```python
from build123d import *

# Parameters (mm, degrees)
F1_DEPTH = 27
F2_W     = 1
F2_H     = 14.5
F2_W_2   = 1.25
F2_H_2   = 3
F2_H_3   = 4.5
F3_DEPTH = 75
F4_R     = 2


with BuildPart() as f1:
    # F0 (on Top) → F1 (new body)
    with BuildSketch(Plane.XY):
        Polygon((10, -5), (27, -5), (27, 5), (-27, 5), (-27, -5), (-10, -5), (-10, -2.5), (10, -2.5), align=None)
    extrude(amount=F1_DEPTH)

    # F2 (on face) → F3 (cut)
    with BuildSketch(Plane(origin=(-27, 0, 0), x_dir=(0, -1, 0), z_dir=(-1, 0, 0))):
        with Locations((-4.5, 12.25)):
            Rectangle(F2_W, F2_H)
        with Locations((-3.375, 12.25)):
            Rectangle(F2_W_2, F2_H)
        with Locations((-4.5, 3.5)):
            Rectangle(F2_W, F2_H_2)
        with Locations((-4.5, 21.75)):
            Rectangle(F2_W, F2_H_3)
    extrude(amount=-F3_DEPTH, mode=Mode.SUBTRACT)

    # F4
    f4_edges = [f1.edges().sort_by_distance(p)[0] for p in [
        (0, 5, 27),
    ]]
    fillet(f4_edges, radius=F4_R)


solid = f1.part
```
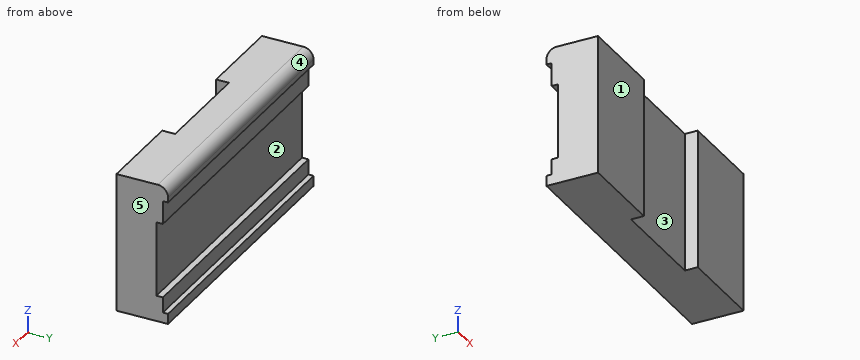
CAD build for the part. Positions are in the model's coordinates, mm. Face numbers are marked on the shaded views. A direction names the side the tool comes from. Round coordinates to 2 decimals unless told otherwise and drop trailing zeros. Order: outer loops, then holes, each group sorted by start corner. A loop starts at its lowest first (then second) coordinate and runs counter-clockwise, first axis right, second up.
Item 1: Saw through at D-D on x = -20.5. Write the cut outline in (y, z), then the cut area to 3 significant figures.
Item 2: Mould opens along X. For the marked faces 3, 4 and 5 say: pulls with the +X half, pulls with the -X half, needs draft (parallel to the pull), parting line crosses it, or undercut.
Item 3: Saw through at B-B on x = -6. Write the cut outline in (y, z), then the cut area to 3 significant figures.
Item 4: Pin check, flat tips, straight feed: pin 1 (0.9 mm diameter, centred on x = -13, z = 3.5, fed in from +Y); pin 2 (0.5 mm diameter, centred on x = 4.5, y = 4.5, fed in from +Z). Stop position of each tip, or through.
Item 5: Saw through at A-A on y = -3.75. Write the cut outline in (x, z).
Item 6: Probe line 1 along Y through (x, z) = (-3.5, 2.5); line 2 along X through (y, z) = (-2.75, 9); line 3 along Y through (x, z) = (-19, 5.75). List the from-to ranges inside material, lowest first.
Item 7: Tool access for the marked faces 1 and 2: list every direction of +Z, -Z, +X, -X, +Y, -Y with a clear straight run to the whole face (end or side of a thin tool).
Item 8: Saw through at C-C on z = 3.5. Write the cut outline in (x, y), then the cut area to 3 significant figures.
Reported:
1. outline: (-5, 0) - (5, 0) - (5, 2) - (4, 2) - (4, 5) - (2.75, 5) - (2.75, 19.5) - (4, 19.5) - (4, 24) - (5, 24) - (5, 25) arc R2 ccw to (3, 27) - (-5, 27) - close
1. area: 229 mm2
2. face 3: undercut
2. face 4: needs draft
2. face 5: pulls with the +X half
3. outline: (-2.5, 0) - (5, 0) - (5, 2) - (4, 2) - (4, 5) - (2.75, 5) - (2.75, 19.5) - (4, 19.5) - (4, 24) - (5, 24) - (5, 25) arc R2 ccw to (3, 27) - (-2.5, 27) - close
3. area: 162 mm2
4. pin 1: stops at y = 4
4. pin 2: stops at z = 26.56
5. outline: (-27, 0) - (-10, 0) - (-10, 27) - (-27, 27) - close; (10, 0) - (27, 0) - (27, 27) - (10, 27) - close
6. line 1: y = -2.5 to 4
6. line 2: x = -27 to -10, 10 to 27
6. line 3: y = -5 to 2.75
7. face 1: +Z, -Z, +X, -X, -Y
7. face 2: +X, -X, +Y
8. outline: (-27, -5) - (-10, -5) - (-10, -2.5) - (10, -2.5) - (10, -5) - (27, -5) - (27, 4) - (-27, 4) - close
8. area: 436 mm2
